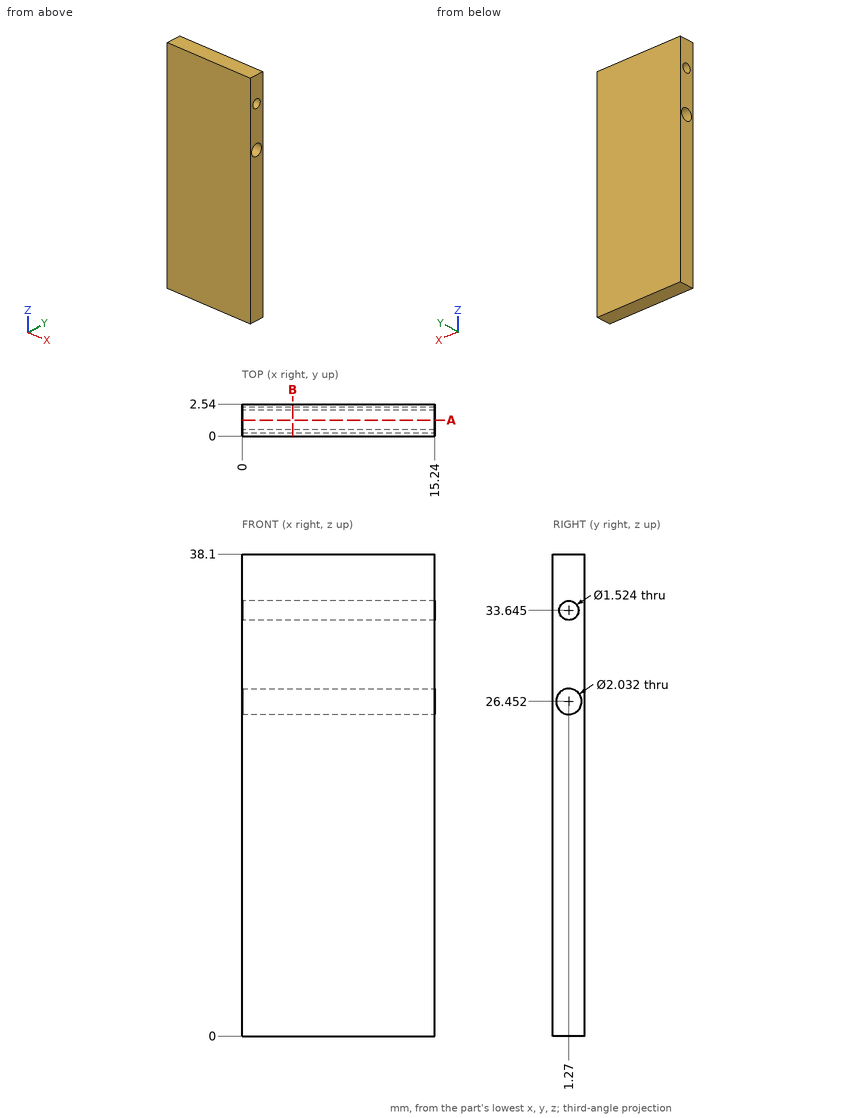
Geometry check sheet. Reference: drawing and pictorial views, mm from the part's lowest x, y, z. Coordinates: 2 decimals unless noted, no trailing zeros. Order: outer loops, then holes, each group sorted by start corner. A loop starts at its lowest first (then second) coordinate and runs counter-clockwise, first axis right, second up.
Item 1: Material ranges on L1, parallel to Z at x = 11, y = 1.27; L2, parallel to Y at x = 14, z = 26.5 (1 decimal); L3, parallel to Z at x = 3.25, y = 1.05 (1 decimal), recorded low to high.
Filled in:
L1: z = 0 to 25.44, 27.47 to 32.88, 34.41 to 38.1
L2: y = 0 to 0.3, 2.3 to 2.5
L3: z = 0 to 25.5, 27.4 to 32.9, 34.4 to 38.1
Item 2: Section check A-A, the plane y = 1.27. Enter the section's corners in (x, z).
Filled in:
outline: (0, 0) - (15.24, 0) - (15.24, 25.44) - (0, 25.44) - close; (0, 27.47) - (15.24, 27.47) - (15.24, 32.88) - (0, 32.88) - close; (0, 34.41) - (15.24, 34.41) - (15.24, 38.1) - (0, 38.1) - close
Item 3: Section check B-B, the plane x = 4. Enter the section's corners in (y, z) (1 decimal).
Filled in:
outline: (0, 0) - (2.5, 0) - (2.5, 38.1) - (0, 38.1) - close; hole circle Ø2 at (1.3, 26.5); hole circle Ø1.5 at (1.3, 33.6)
